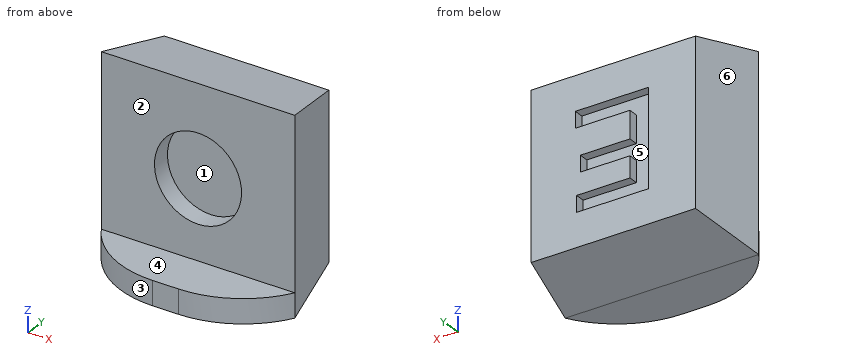
from build123d import *

# Parameters (mm, degrees)
SKETCH1_W               = 8
SKETCH1_H               = 8
BOSS_EXTRUDE1_DEPTH     = 3
CUT_EXTRUDE1_DEPTH      = 12.704699911
CUT_EXTRUDE1_DEPTH_BACK = 12.704699911
CUT_EXTRUDE2_DEPTH      = 11
SKETCH4_R               = 1.8
CUT_EXTRUDE3_DEPTH      = 0.8
SKETCH5_W               = 8
SKETCH5_H               = 1
BOSS_EXTRUDE2_DEPTH     = 2
FILLET1_R               = 4
CUT_EXTRUDE4_DEPTH      = 0.4


with BuildPart() as part:
    # Sketch1 → Boss-Extrude1 (new body)
    with BuildSketch(Plane(origin=(0, 0, 0), x_dir=(1, 0, 0), z_dir=(0, 1, 0))):
        with Locations((4, 4)):
            Rectangle(SKETCH1_W, SKETCH1_H)
    extrude(amount=BOSS_EXTRUDE1_DEPTH)

    # Sketch2 → Cut-Extrude1 (cut, two sides: drawn at the far end of the back side and taken through both)
    with BuildSketch(Plane.XY.offset(-CUT_EXTRUDE1_DEPTH_BACK)):
        Polygon((0, 0), (0.6, 3), (0, 3), align=None)
        Polygon((8, 0), (7.4, 3), (8, 3), align=None)
    extrude(amount=CUT_EXTRUDE1_DEPTH + CUT_EXTRUDE1_DEPTH_BACK, mode=Mode.SUBTRACT)

    # Sketch3 → Cut-Extrude2 (cut)
    with BuildSketch(Plane(origin=(0, 0, 0), x_dir=(0, 0, -1), z_dir=(1, 0, 0))):
        Polygon((0, 0), (0.6, 3), (0, 3), align=None)
        Polygon((8, 3), (7.4, 3), (8, 0), align=None)
    extrude(amount=CUT_EXTRUDE2_DEPTH, mode=Mode.SUBTRACT)

    # Sketch4 → Cut-Extrude3 (cut)
    with BuildSketch(Plane.XZ):
        with Locations(Location((4, -3.75, 0), (0, 0, 270))):
            Circle(SKETCH4_R)
    extrude(amount=-CUT_EXTRUDE3_DEPTH, mode=Mode.SUBTRACT)

    # Sketch5 → Boss-Extrude2 (add)
    with BuildSketch(Plane.XZ):
        with Locations((4, -7.5)):
            Rectangle(SKETCH5_W, SKETCH5_H)
    extrude(amount=BOSS_EXTRUDE2_DEPTH)

    # Fillet1
    # the kernel refuses this fillet: 4 mm, written as the material it takes off along each edge
    with BuildSketch(Plane(origin=(8, -2, -16.660254038), x_dir=(0, 1, 0), z_dir=(0, 0, 1)), Plane(origin=(0, -2, 1.660254038), x_dir=(0, 1, 0), z_dir=(0, 0, -1))) as fillet1_piece_1:
        with BuildLine():
            CenterArc((4, 3.464101615), FILLET1_R, 180, 60)
            Line((0, 3.464101615), (-0.08, 3.464101615))
            Line((-0.08, 3.464101615), (-0.08, 0))
            Line((-0.08, 0), (0, -0.08))
            ThreePointArc((0, -0.08), (1, -0.08), (1.96, -0.069282032))
            Line((1.96, -0.069282032), (2, 0))
        make_face()
    extrude(amount=18.320508076, mode=Mode.SUBTRACT)

    # Sketch6 → Cut-Extrude4 (cut)
    with BuildSketch(Plane(origin=(0, 3, 0), x_dir=(1, 0, 0), z_dir=(0, 1, 0))):
        Polygon((2.544225106, 2.010567225), (2.544225106, 6.010567225), (5.51858408, 6.010567225), (5.51858408, 5.343900558), (3.313455875, 5.343900558), (3.313455875, 4.472105686), (5.364737926, 4.472105686), (5.364737926, 3.80543902), (3.313455875, 3.80543902), (3.313455875, 2.677233891), (5.569866131, 2.677233891), (5.569866131, 2.010567225), align=None)
    extrude(amount=-CUT_EXTRUDE4_DEPTH, mode=Mode.SUBTRACT)


solid = part.part
Geometry check sheet. Reference: the model listing, model coordinates, mm. Face numbers are marked on the shaded views. A direction names the side the tool comes from. Round coordinates to 2 decimals unless told otherwise and drop trailing zeros. Order: outer loops, then holes, each group sorted by start corner. A loop starts at its lowest first (then second) coordinate and runs counter-clockwise, first axis right, second up. Notation, with made-up numbers: M 64,-9.75 L 107,-9.75 A19 ccw 107,19.25 Z; hole C 15,63.25 d4. An arc over 180 degrees is marked long. Answer in a Markdown table with one row per item. Add a question column.
Item 1: Set-up check for the marked faces 1, 2 and 3: record each of +Z, -Z, +X, -X, +Y, -Y from which the full face is reachable in a straight line by a thin tool's end or side.
Item 2: Sectioned sample at C-C, the plane z = -4.75. Enter the section's corners in (x, y).
Item 3: Draft check along Z on the marked faces 4, 5 and 6. Enter one of: released by +Z, released by -Z, zero draft, split by the parting line, or undercut.
Item 4: Material ranges on L1, parallel to Z at x = 5, y = -0.1; L2, parallel to Y at x = 1.5, z = -6.5; L3, parallel to X at y = 0.25, z = -3.75, recorded low to high. Write a range as [from, to].
Item 5: Depth check by flat-ended pin: pin 1 Ø1.5 at (x, y) = (3.5, -1) entering from +Z; pin 2 Ø2 at (x, z) = (3, -5.5) entering from -Y; pin 3 Ø3 at (x, y) = (7, 2) entering from +Z. Enter the tip coordinate at first touch or a pass-through.
Item 6: Sectioned sample at B-B, the plane x = 4. Enter the section's corners in (y, z), plus the area to 3 significant figures.
Item 7: Sectioned sample at A-A, the plane y = 0.1. Enter the section's corners in (x, z), plus the area to 3 significant figures.
Item 8: Sectioned sample at D-D, the plane y = 1.1. Enter the section's corners in (x, z), plus the area to 3 significant figures.
Filled in:
| question | item | result |
|---|---|---|
| 1 | face 1 | -Y |
| 1 | face 2 | +Z, +X, -X, -Y |
| 1 | face 3 | +Z, -Z, -X, -Y |
| 2 | outline | M 0,0 L 2.5,0 L 2.5,0.8 L 5.5,0.8 L 5.5,0 L 8,0 L 7.4,3 L 3.31,3 L 3.31,2.6 L 2.54,2.6 L 2.54,3 L 0.6,3 Z |
| 3 | face 4 | released by +Z |
| 3 | face 5 | undercut |
| 3 | face 6 | zero draft |
| 4 | L1 | z = [-8, -7] |
| 4 | L2 | y = [0, 3] |
| 4 | L3 | x = [0.05, 2.2], [5.8, 7.95] |
| 5 | pin 1 | stops at z = -7 |
| 5 | pin 2 | stops at y = 0 |
| 5 | pin 3 | stops at z = -0.1 |
| 6 | outline | M -2,-8 L 0,-8 L 3,-7.4 L 3,-6.01 L 2.6,-6.01 L 2.6,-5.34 L 3,-5.34 L 3,-4.47 L 2.6,-4.47 L 2.6,-3.81 L 3,-3.81 L 3,-2.68 L 2.6,-2.68 L 2.6,-2.01 L 3,-2.01 L 3,-0.6 L 0,0 L 0,-1.95 L 0.8,-1.95 L 0.8,-5.55 L 0,-5.55 L 0,-7 L -2,-7 Z |
| 6 | area | 20.5 mm² |
| 7 | outline | M 0.02,-7.98 L 7.98,-7.98 L 7.98,-0.02 L 0.02,-0.02 Z; hole C 4,-3.75 d3.6 |
| 7 | area | 53.2 mm² |
| 8 | outline | M 0.22,-7.78 L 7.78,-7.78 L 7.78,-0.22 L 0.22,-0.22 Z |
| 8 | area | 57.2 mm² |
